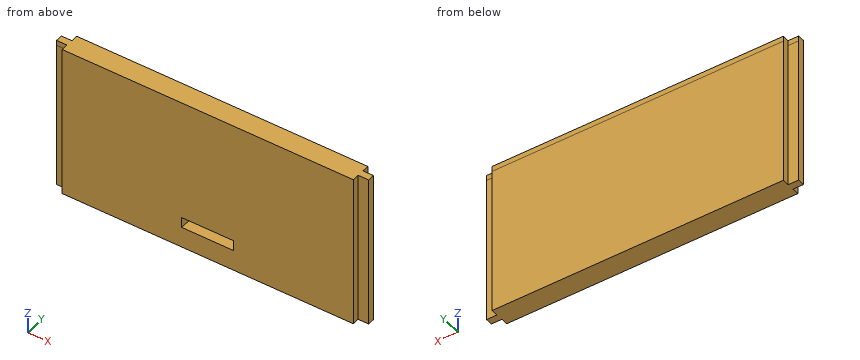
```python
from build123d import *

# Parameters (mm, degrees)
PAD015_DEPTH    = 28.35
POCKET020_DEPTH = 2
PAD045_DEPTH    = 1


with BuildPart() as part:
    # Sketch029 → Pad015 (new body)
    with BuildSketch(Plane.XY):
        Polygon((-78.25, -81.000001), (-78.25, -82.333334), (-80.25, -82.333334), (-80.25, -83.666667), (-78.25, -83.666667), (-78.25, -85), (-22.25, -85), (-22.25, -83.666667), (-20.25, -83.666667), (-20.25, -82.333334), (-22.25, -82.333334), (-22.25, -81.000001), align=None)
    extrude(amount=PAD015_DEPTH)

    # Sketch037 (on Face6 of Pad015) → Pocket020 (cut)
    with BuildSketch(Plane.XZ.offset(85)):
        Polygon((-55.25, 6), (-45.25, 6), (-45.25, 4), (-50.25, 4), (-55.25, 4), align=None)
    extrude(amount=-POCKET020_DEPTH, mode=Mode.SUBTRACT)

    # Pocket020 Face5 → Pad045 (add)
    with BuildSketch(Plane(origin=(-50.25, -83, 28.35), x_dir=(0, 1, 0), z_dir=(0, 0, 1))):
        Polygon((2, 28), (0.666667, 28), (0.666667, 30), (-0.666666, 30), (-0.666666, 28), (-2, 28), (-2, -28), (-0.666667, -28), (-0.666667, -30), (0.666667, -30), (0.666667, -28), (2, -28), align=None)
    extrude(amount=PAD045_DEPTH)


with BuildPart() as part_1:
    # Body003 placement: moved
    add(part.part.moved(Location((0, -20, -56))))


solid = part_1.part
```
Geometry check sheet. Reference: the model listing, model coordinates, mm. Coordinates: 2 decimals unless noted, no trailing zeros. Order: outer loops, then holes, each group sorted by start corner. A loop starts at its lowest first (then second) coordinate and runs counter-clockwise, first axis right, second up. Notation, with made-up numbers: (48, 44.5) - (91, 44.5) arc R32 cw to (91, 79.5) - close; hole circle Ø10 at (5, -11). An arc over 180 degrees is marked (long way). Answer in a Markdown table with one row per item. Add a question column.
1. Section check A-A (z = -39.75). Enter the section's corners in (x, y), plus the area to 3 significant figures.
2. Material ranges on L1, parallel to X at y = -103.6, z = -51.75; L2, parallel to X at y = -104.8, z = -33.5; L3, parallel to Z at x = -47, y = -103.4, recorded low to high. Write a range as [from, to].
3. Gauge pin test, flat ends, axial feed: pin 1 Ø0.6 at (x, z) = (-21, -47.5) entering from -Y; pin 2 Ø1.1 at (x, z) = (-21, -27) entering from +Y; pin 3 Ø1.1 at (y, z) = (-101.5, -40.5) entering from -X. Record the tip position at first contact, or that the pin passes through.
Data:
| question | item | result |
|---|---|---|
| 1 | outline | (-80.25, -103.67) - (-78.25, -103.67) - (-78.25, -105) - (-22.25, -105) - (-22.25, -103.67) - (-20.25, -103.67) - (-20.25, -102.33) - (-22.25, -102.33) - (-22.25, -101) - (-78.25, -101) - (-78.25, -102.33) - (-80.25, -102.33) - close |
| 1 | area | 229 mm² |
| 2 | L1 | x = [-80.25, -55.25], [-45.25, -20.25] |
| 2 | L2 | x = [-78.25, -22.25] |
| 2 | L3 | z = [-56, -52], [-50, -26.65] |
| 3 | pin 1 | stops at y = -103.67 |
| 3 | pin 2 | stops at y = -102.33 |
| 3 | pin 3 | stops at x = -78.25 |
